Geometry: final body of the model. Coordinates: model frame, mm. Face numbers are marked on the shaded views. A direction names the side the tool comes from. Coordinates: 2 decimals unless noted, no trailing zeros. Order: outer loops, then holes, each group sorted by start corner. A loop starts at its lowest first (then second) coordinate and runs counter-clockwise, first axis right, second up. Notation, with made-up numbers: M 74.25,35 L 82.25,35 A26 ccw 82.25,57 Z; hole C 64,-14 d4. An arc over 180 degrees is marked long. Write item = value, one per line. Start each with the question number.
```python
from build123d import *

# Parameters (mm, degrees)
SKETCH1_R           = 8
BOSS_EXTRUDE1_DEPTH = 450
SKETCH2_W           = 40
SKETCH2_H           = 52
BOSS_EXTRUDE2_DEPTH = 20
CHAMFER1_SIZE       = 12
SKETCH3_R           = 2.5
CUT_EXTRUDE1_DEPTH  = 10


with BuildPart() as part:
    # Sketch1 → Boss-Extrude1 (new body)
    with BuildSketch(Plane(origin=(0, 0, 0), x_dir=(0, 0, -1), z_dir=(1, 0, 0))):
        Circle(SKETCH1_R)
    extrude(amount=BOSS_EXTRUDE1_DEPTH)

    # Sketch2 → Boss-Extrude2 (add, symmetric)
    with BuildSketch(Plane(origin=(0, 0, 0), x_dir=(1, 0, 0), z_dir=(0, 1, 0))):
        with Locations((200, 0)):
            Rectangle(SKETCH2_W, SKETCH2_H)
    extrude(amount=BOSS_EXTRUDE2_DEPTH, both=True)

    # Chamfer1
    chamfer1_edges = [part.edges().sort_by_distance(p)[0] for p in [
        (200, -20, 26),
        (200, -20, -26),
    ]]
    chamfer(chamfer1_edges, length=CHAMFER1_SIZE)

    # Sketch3 → Cut-Extrude1 (cut)
    with BuildSketch(Plane(origin=(0, 20, 0), x_dir=(1, 0, 0), z_dir=(0, 1, 0))):
        with Locations((188, 20)):
            Circle(SKETCH3_R)
        with Locations((212, 20)):
            Circle(SKETCH3_R)
        with Locations((188, -20)):
            Circle(SKETCH3_R)
        with Locations((212, -20)):
            Circle(SKETCH3_R)
    extrude(amount=-CUT_EXTRUDE1_DEPTH, mode=Mode.SUBTRACT)


solid = part.part
```
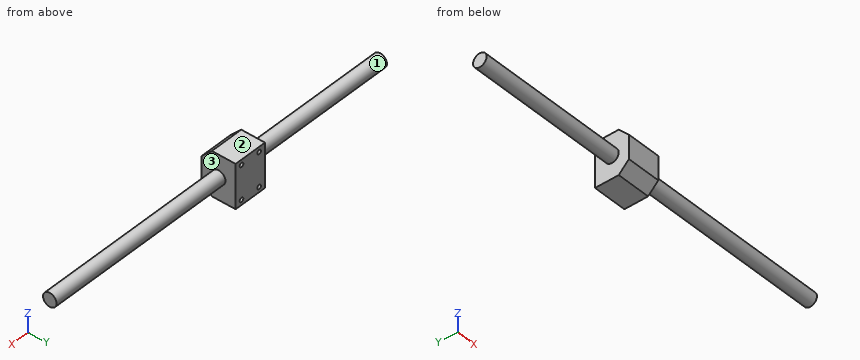
Item 1: Section query C-C on x = 228. Output: boundary loops of the cut face in (y, z), and give its area (3 significant figures).
Item 2: Section query D-D on y = -15. Output: boundary loops of the cut face in (x, z).
Item 3: Section query A-A on y = 14. Output: boundary loops of the cut face in (x, z).
Item 4: First-contact query: pin 1 (10 mm diameter, centred on x = 287.5, y = -13.5, fed in from -Z); pin 2 (2.5 mm diameter, centred on x = 212.5, z = 20.5, fed in from +Y); pin 3 (12 mm diameter, centred on x = 343.5, y = -10.5, fed in from -Z); pin 4 (10 mm diameter, centred on x = 284.5, y = -4.5, fed in from -Z). Flat tips, straight axial feed; report the tip coordinate or a pass-through.
Item 5: Reachability of the marked faces 1, 2 and 3 from +Z, -Z, +X, -X, +Y, -Y: full face, straight path, thin tool, end or side. Return the list, or none.
Item 6: Material intervals for probe 1 along Z at (x, y) = (212, 16.5); probe 2 along X at (y, z) = (14, -20); probe 3 along Z at (x, y) = (210, 15), sorted ascending. Write a range as [from, to].
Item 7: Section query B-B on z = 0. Output: boundary loops of the cut face in (x, y), and give its area (3 significant figures).
Ans:
q1.outline = C 0,0 d16
q1.area = 201 mm^2
q2.outline = M 180,-19 L 220,-19 L 220,19 L 180,19 Z
q3.outline = M 180,-26 L 220,-26 L 220,26 L 180,26 Z; hole C 188,-20 d5; hole C 188,20 d5; hole C 212,-20 d5; hole C 212,20 d5
q4.pin_1 = through
q4.pin_2 = 10
q4.pin_3 = -6.61
q4.pin_4 = -8
q5.face_1 = -X
q5.face_2 = +Z, +X, -X, +Y, -Y
q5.face_3 = +X
q6.probe_1 = [-26, -22.5], [-17.5, 17.5], [22.5, 26]
q6.probe_2 = [180, 185.5], [190.5, 209.5], [214.5, 220]
q6.probe_3 = [-26, -21.5], [-18.5, 18.5], [21.5, 26]
q7.outline = M 0,-8 L 180,-8 L 180,-20 L 220,-20 L 220,-8 L 450,-8 L 450,8 L 220,8 L 220,20 L 180,20 L 180,8 L 0,8 Z
q7.area = 8,160 mm^2
